```python
from build123d import *

# Parameters (mm, degrees)
SKETCH_1_W          = 20
SKETCH_1_H          = 20
EXTRUDE_1_DEPTH     = 50
CUT_EXTRUDE_1_DEPTH = 50


with BuildPart() as part:
    # 草圖1 → 填料-伸長1 (new body)
    with BuildSketch(Plane.XY):
        Rectangle(SKETCH_1_W, SKETCH_1_H)
    extrude(amount=EXTRUDE_1_DEPTH)

    # 草圖2 → 除料-伸長1 (cut)
    with BuildSketch(Plane.XY):
        with BuildLine():
            Line((-4, 5), (4, 5))
            ThreePointArc((4, 5), (6, 0), (4, -5))
            Line((4, -5), (-4, -5))
            ThreePointArc((-4, -5), (-6, 0), (-4, 5))
        make_face()
    extrude(amount=CUT_EXTRUDE_1_DEPTH, mode=Mode.SUBTRACT)


solid = part.part
```
Work out the finished part from the listing and answer in its coordinate system (mm). A direction names the side the tool comes from. Give positions to 0.01 mm unless a question says otherwise; leave off trailing zeros. Order: outer loops, then holes, each group sorted by start corner. A loop starts at its lowest first (then second) coordinate and runs counter-clockwise, first axis right, second up. Notation, with made-up numbers: (84, 43.5) - (90, 43.5) arc R20 ccw to (90, 62.5) - close; hole circle Ø3 at (-27.5, 68). An arc over 180 degrees is marked (long way). One line per item, written item: value. Start each with the question number.
1. Consider line 1 (Y direction, x = -1.25, z = 27.5); line 2 (X direction, y = 0.25, z = 33); line 3 (Y direction, x = -5, z = 29). Determine where each line is inside the solid, lowest interval first.
2. For a pull along X with two mould halves and no side action, classify faces 1 (the face through (0, -10, 25)), 2 (the face through (0, -5, 25)), 3 (the face through (10, 0, 25)) as released by +X, released by -X, zero draft, split by the parting line, or undercut.
3. Section B-B, the plane z = 32 is taken. Write down the section's boundary in (x, y).
4. This flat-tipped pin is pushed along its axis until it touches: pin 1 Ø12 at (x, y) = (-5.5, 5.5) entering from -Z. Where does it stop, or does it pass through?
5. Section C-C, the plane y = -0.25 is taken. Write down the section's boundary in (x, z), then the cut area to 3 significant figures.
6. Section A-A, the plane x = 2.5 is taken. Write down the section's boundary in (y, z), then the cut area to 3 significant figures.
7. Which of the six approach directions +Z, -Z, +X, -X, +Y, -Y give full straight-line access (tool end or side, diameter ignored) to faces 4 (the face through (-6, 0, 25)), 5 (the face through (-5, 5, 50))?
Filled sheet:
1. line 1: -10 to -5, 5 to 10
1. line 2: -10 to -6, 6 to 10
1. line 3: -10 to -3.67, 3.67 to 10
2. face 1: zero draft
2. face 2: undercut
2. face 3: released by +X
3. outline: (-10, -10) - (10, -10) - (10, 10) - (-10, 10) - close; hole (-4, -5) - (4, -5) arc R7.25 ccw to (4, 5) - (-4, 5) arc R7.25 ccw to start
4. pin 1: z = 0
5. outline: (-10, 0) - (-6, 0) - (-6, 50) - (-10, 50) - close; (6, 0) - (10, 0) - (10, 50) - (6, 50) - close
5. area: 400 mm²
6. outline: (-10, 0) - (-5, 0) - (-5, 50) - (-10, 50) - close; (5, 0) - (10, 0) - (10, 50) - (5, 50) - close
6. area: 500 mm²
7. face 4: +Z, -Z
7. face 5: +Z, +X, -X, +Y, -Y
